from build123d import *

# Parameters (mm, degrees)
SKETCH1_W     = 6.5
SKETCH1_H     = 7
CHAMFER1_SIZE = 0.1


with BuildPart() as part:
    # Sketch1 → Revolve1 (revolve)
    with BuildSketch(Plane(origin=(0, 0, 0), x_dir=(0, 0, -1), z_dir=(1, 0, 0))):
        with Locations((30.75, 0)):
            Rectangle(SKETCH1_W, SKETCH1_H)
    revolve(axis=Axis((0, 3.5, 0), (0, -1, 0)))

    # Sketch3 → Cut-Revolve2 (revolve, cut)
    with BuildSketch(Plane(origin=(0, 0, 0), x_dir=(0, 0, -1), z_dir=(1, 0, 0))):
        Polygon((31.8, 3.3), (32, 3.1), (32, 3.5), (29.5, 3.5), (29.5, 3.1), (29.7, 3.3), align=None)
    cut_revolve2 = revolve(axis=Axis((0, 3.5, 0), (0, -1, 0)), mode=Mode.SUBTRACT)

    # Mirror1: Cut-Revolve2 across plane
    add(cut_revolve2.mirror(Plane.ZX), mode=Mode.SUBTRACT)

    # Chamfer1
    chamfer1_edges = [part.edges().sort_by_distance(p)[0] for p in [
        (0, 3.5, 32),
        (0, 3.5, 29.5),
        (0, -3.5, 32),
        (0, -3.5, 29.5),
        (0, 3.5, 34),
        (0, -3.5, 34),
        (0, -3.5, 27.5),
        (0, 3.5, 27.5),
    ]]
    chamfer(chamfer1_edges, length=CHAMFER1_SIZE)


solid = part.part
Verification items for the finished model (mm, model axes). A direction names the side the tool comes from. Coordinates: 2 decimals unless noted, no trailing zeros. Write each loop counter-clockwise with the first axis right and the second up, starting at its lowest first coordinate (ties: lowest second). Pieces come first, ordered by that corner, then holes. Notation, with made-up numbers: M -23.75,9.5 L -14.75,9.5 A16 ccw -14.75,38.5 Z; hole C -40,25.5 d3. An arc over 180 degrees is marked long. One line per question, with ' | ' between items.
1) Material ranges on L1, parallel to X at y = 3.35, z = 0; L2, parallel to X at y = 0.75, z = 0; L3, parallel to Y at x = 31.5, z = 1.5, recorded low to high.
Solutions:
L1: -34 to -32, -29.5 to -27.5, 27.5 to 29.5, 32 to 34 | L2: -34 to -27.5, 27.5 to 34 | L3: -3.3 to 3.3
2) Sectioned sample at A-A on y = 1.5. Record the cut outline in (x, z), then the cut area to 3 significant figures.
Solutions:
outline: C 0,0 d68; hole C 0,0 d55 | area: 1,260 mm^2
3) Depth check by flat-ended pin: pin 1 Ø1.5 at (x, y) = (-4.5, 1) entering from -Z; pin 2 Ø2 at (x, y) = (-9, 0) entering from -Z; pin 3 Ø1 at (x, y) = (9, -1.5) entering from -Z. Enter the tip coordinate at first touch or a pass-through.
Solutions:
pin 1: z = -33.79 | pin 2: z = -33.05 | pin 3: z = -32.92
4) Access from +Z, -Z, +X, -X, +Y, -Y to the whole of each face (thin tool, end or side, straight path). Record for faces 1 (the face through (28.4, 3.3, 9.3)), 2 (the face through (-12, -3.5, 30)).
Solutions:
face 1: +Y | face 2: +Z, -Z, +X, -X, -Y
